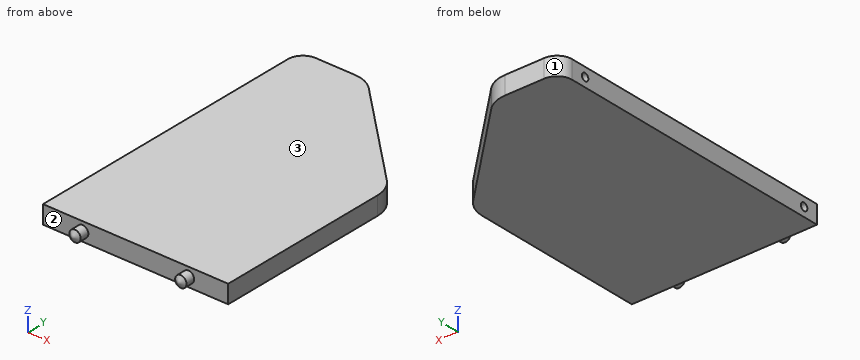
```python
from build123d import *

# Parameters (mm, degrees)
SKETCH4_W                    = 122.5
SKETCH4_H                    = 200
BOSS_EXTRUDE1_DEPTH          = 12
CUT_EXTRUDE1_DEPTH           = 12
FILLET1_R                    = 20
FILLET2_R                    = 20
FILLET3_R                    = 10
SKETCH10_R                   = 3.75
BOSS_EXTRUDE3_DEPTH          = 6
F_5_0_5_DIAMETER_HOLE1_D     = 5
F_5_0_5_DIAMETER_HOLE1_DEPTH = 8
F_5_0_5_DIAMETER_HOLE1_TIP   = 1.502151548
F_5_0_5_DIAMETER_HOLE2_D     = 5
F_5_0_5_DIAMETER_HOLE2_DEPTH = 8
F_5_0_5_DIAMETER_HOLE2_TIP   = 1.502151548
SCALE1_SCALE                 = 0.9


with BuildPart() as part:
    # Sketch4 → Boss-Extrude1 (new body)
    with BuildSketch(Plane.XY):
        with Locations((61.25, 100)):
            Rectangle(SKETCH4_W, SKETCH4_H)
    extrude(amount=BOSS_EXTRUDE1_DEPTH)

    # Sketch7 → Cut-Extrude1 (cut)
    with BuildSketch(Plane.XY.offset(12)):
        Polygon((43.985796602, 200), (122.5, 124.415794753), (122.5, 200), align=None)
    extrude(amount=-CUT_EXTRUDE1_DEPTH, mode=Mode.SUBTRACT)

    # Fillet1
    fillet1_edges = [part.edges().sort_by_distance(p)[0] for p in [
        (43.985796602, 200, 6),
    ]]
    fillet(fillet1_edges, radius=FILLET1_R)

    # Fillet2
    fillet2_edges = [part.edges().sort_by_distance(p)[0] for p in [
        (122.5, 124.415794753, 6),
    ]]
    fillet(fillet2_edges, radius=FILLET2_R)

    # Fillet3
    fillet3_edges = [part.edges().sort_by_distance(p)[0] for p in [
        (0, 200, 6),
    ]]
    fillet(fillet3_edges, radius=FILLET3_R)

    # Sketch10 → Boss-Extrude3 (add)
    with BuildSketch(Plane.XZ):
        with Locations(Location((26.25, 6, 0), (0, 0, 90))):
            Circle(SKETCH10_R)
        with Locations(Location((96.25, 6, 0), (0, 0, 90))):
            Circle(SKETCH10_R)
    extrude(amount=BOSS_EXTRUDE3_DEPTH)

    # Boss-Extrude4 cone 1 section (through the dimple's axis) → Boss-Extrude4 (revolve)
    with BuildSketch(Plane(origin=(26.25, -6, 6), x_dir=(0, 0, 1), z_dir=(1, 0, 0))):
        Polygon((0, 0), (3.75, 0), (0, 1.993910369), align=None)
    revolve(axis=Axis((26.25, -6, 6), (0, -1, 0)))

    # Boss-Extrude4 cone 2 section (through the dimple's axis) → Boss-Extrude4 cone 2 (revolve)
    with BuildSketch(Plane(origin=(96.25, -6, 6), x_dir=(0, 0, 1), z_dir=(1, 0, 0))):
        Polygon((0, 0), (3.75, 0), (0, 1.993910369), align=None)
    revolve(axis=Axis((96.25, -6, 6), (0, -1, 0)))

    # Ø5.0 (5) Diameter Hole1
    with Locations(Plane.ZY):
        with Locations((6, 180)):
            Hole(F_5_0_5_DIAMETER_HOLE1_D / 2, depth=F_5_0_5_DIAMETER_HOLE1_DEPTH)
            with Locations((0, 0, -(F_5_0_5_DIAMETER_HOLE1_DEPTH + F_5_0_5_DIAMETER_HOLE1_TIP / 2))):  # 118° drill point
                Cone(0, F_5_0_5_DIAMETER_HOLE1_D / 2, F_5_0_5_DIAMETER_HOLE1_TIP, mode=Mode.SUBTRACT)

    # Ø5.0 (5) Diameter Hole2
    with Locations(Plane.ZY):
        with Locations((6, 10)):
            Hole(F_5_0_5_DIAMETER_HOLE2_D / 2, depth=F_5_0_5_DIAMETER_HOLE2_DEPTH)
            with Locations((0, 0, -(F_5_0_5_DIAMETER_HOLE2_DEPTH + F_5_0_5_DIAMETER_HOLE2_TIP / 2))):  # 118° drill point
                Cone(0, F_5_0_5_DIAMETER_HOLE2_D / 2, F_5_0_5_DIAMETER_HOLE2_TIP, mode=Mode.SUBTRACT)


with BuildPart() as part_1:
    # Scale1: scaled about (56.525506998, 89.309787592, 6)
    add(part.part.scale(SCALE1_SCALE).moved(Location((5.6525507, 8.930978759, 0.6))))


solid = part_1.part
```
The model under review builds one solid part; all positions refer to its coordinate system, in mm. Face numbers are marked on the shaded views. Round coordinates to 2 decimals unless told otherwise and drop trailing zeros. Loops run counter-clockwise (first coordinate to the right, second up) from the corner with the lowest first, then second, coordinate; pieces in that order, holes last. Notation, with made-up numbers: (36.25, -22) - (81.25, -22) arc R23 cw to (81.25, 14) - close; hole circle Ø2 at (69.5, 55.25). An arc over 180 degrees is marked (long way). Write each question's results on one line, items separated by ' | '. Start each with the question number.
Q1. Take a section at A-A on x = 22. Give the boundary of the cut face in (y, z).
Q2. Take a section at B-B on y = 128. Give the boundary of the cut face in (x, z).
Q3. Wall thickness on line 1 along Y through (x, z) = (9.25, 6); line 2 along Y through (x, z) = (11, 6); line 3 along Y through (x, z) = (19.5, 7): over which ranges is each line inside the solid? List them lowest first. Write a range as [from, to].
Q4. Insertion check: P1, Ø1, axis at x = 39.5, z = 10, coming from the -Y side; P2, Ø6, axis at y = 170.93, z = 6, coming from the +X side; P3, Ø6, axis at x = 68, z = 8.5, coming from the +Y side. Each pin has a flat end and moves straight along its axis. Give the tip position at first contact, or say it passes through.
Q5. Draft analysis for pull direction X (two halves, no side actions). For the marked faces 1, 2 and 3, state which applies: pulls with the +X half, pulls with the -X half, needs draft (parallel to the pull), parting line crosses it, or undercut.
Data:
1) outline: (8.93, 0.6) - (188.93, 0.6) - (188.93, 11.4) - (8.93, 11.4) - close
2) outline: (5.65, 0.6) - (108.53, 0.6) - (108.53, 11.4) - (5.65, 11.4) - close
3) line 1: y = [8.93, 15.68], [20.18, 168.68], [173.18, 187.13] | line 2: y = [8.93, 15.68], [20.18, 168.68], [173.18, 188.16] | line 3: y = [8.93, 188.93]
4) P1: stops at y = 8.93 | P2: stops at x = 67.05 | P3: stops at y = 169.91
5) face 1: pulls with the -X half | face 2: undercut | face 3: needs draft
